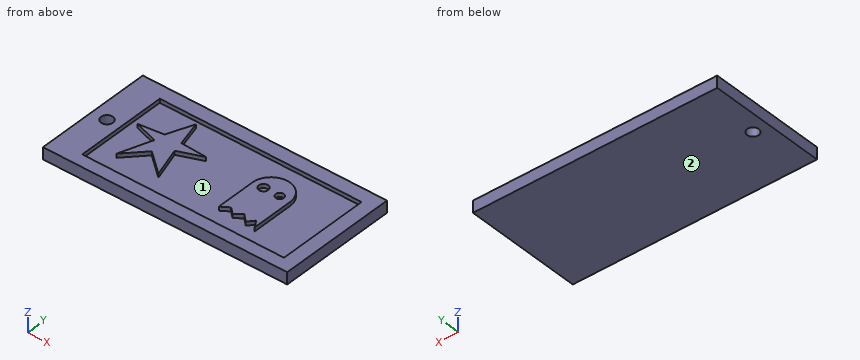
from build123d import *

# Parameters (mm, degrees)
SKETCH_W        = 62
SKETCH_H        = 30
PAD_DEPTH       = 3
SKETCH001_W     = 51.222641
SKETCH001_H     = 23.315135
POCKET_DEPTH    = 1
SKETCH002_R     = 1.5
POCKET001_DEPTH = 3.001
PAD001_DEPTH    = 1
PAD002_DEPTH    = 1
SKETCH005_R     = 1.199553
SKETCH005_R_2   = 1.016367
POCKET002_DEPTH = 1


with BuildPart() as part:
    # Sketch → Pad (new body)
    with BuildSketch(Plane.XY):
        with Locations((-1.286613, 0.704456)):
            Rectangle(SKETCH_W, SKETCH_H)
    extrude(amount=PAD_DEPTH)

    # Sketch001 → Pocket (cut)
    with BuildSketch(Plane.XY.offset(3)):
        with Locations((0.632324, 0.504924)):
            Rectangle(SKETCH001_W, SKETCH001_H)
    extrude(amount=-POCKET_DEPTH, mode=Mode.SUBTRACT)

    # Sketch002 → Pocket001 (cut, through all)
    with BuildSketch(Plane.XY.offset(3)):
        with Locations((-28.453762, 0.41293)):
            Circle(SKETCH002_R)
    extrude(amount=-POCKET001_DEPTH, mode=Mode.SUBTRACT)

    # Sketch003 → Pad001 (new body)
    with BuildSketch(Plane.XY.offset(2)):
        Polygon((-16.856503, 3.99872), (-14.349889, 10.458068), (-12.61454, 3.99872), (-6.058784, 3.709493), (-12.036091, 1.299289), (-9.722297, -6.316956), (-15.313969, -1.689364), (-20.03797, -6.70259), (-17.242132, 1.395697), (-23.123034, 3.227453), align=None)
    extrude(amount=PAD001_DEPTH)

    # Sketch004 → Pad002 (new body)
    with BuildSketch(Plane.XY.offset(2)):
        with BuildLine():
            Line((6.033253, 3.5701), (6.033253, -6.826028))
            Line((6.033253, -6.826028), (8.010232, -5.476315))
            Line((8.010232, -5.476315), (9.649171, -6.922436))
            Line((9.649171, -6.922436), (11.384521, -5.476315))
            Line((11.384521, -5.476315), (13.119864, -7.115253))
            Line((13.119864, -7.115253), (14.469583, -5.572722))
            Line((14.469583, -5.572722), (15.636065, -7.404478))
            Line((15.636065, -7.404478), (15.636065, 3.375676))
            ThreePointArc((15.636065, 3.375676), (10.927253, 8.046213), (6.033253, 3.5701))
        make_face()
    extrude(amount=PAD002_DEPTH)

    # Sketch005 → Pocket002 (cut)
    with BuildSketch(Plane.XY.offset(3)):
        with Locations((8.755972, 3.403389)):
            Circle(SKETCH005_R)
        with Locations((12.882946, 3.403389)):
            Circle(SKETCH005_R_2)
    extrude(amount=-POCKET002_DEPTH, mode=Mode.SUBTRACT)


solid = part.part
The model under review builds one solid part; all positions refer to its coordinate system, in mm. Face numbers are marked on the shaded views. Give positions to 0.01 mm unless a question says otherwise; leave off trailing zeros. Order: outer loops, then holes, each group sorted by start corner. A loop starts at its lowest first (then second) coordinate and runs counter-clockwise, first axis right, second up. Notation, with made-up numbers: M 74,-31 L 86,-31 A27 ccw 86,6 Z; hole C 88,46.25 d11. An arc over 180 degrees is marked long. Answer in a Markdown table with one row per item. Add a question column.
1. Add section C-C on x = 19.5. State the section outline as (y, z) points, plus the area to 3 significant figures.
2. Add section B-B on y = -10. State the section outline as (x, z) points, plus the area to 3 significant figures.
3. Mouldability with a two-part tool opening along X and no side actions: class the marked faces 1 and 2 as released by +X, released by -X, zero draft, split by the parting line, or undercut.
4. For pin 1 Ø1.4 at (x, y) = (8.76, 3.4) entering from +Z, flat-tipped, find the tip position at first contact; note if it passes through.
5. Add section D-D on y = 9. State the section outline as (x, z) points.
6. To check wall thickness, follow line 1 along Y through (x, z) = (22, 2.5); line 2 along Y through (x, z) = (13, 2.05); line 3 along X through (y, z) = (-0.25, 2.15). State the ranges of each line that lie inside material, in increasing order.
7. Add section A-A on z = 2.45. Count the separate pieces of the cut face and the enclosed holes in it, plus the area to 3 significant figures.
The answers:
| question | item | result |
|---|---|---|
| 1 | outline | M -14.3,0 L 15.7,0 L 15.7,3 L 12.16,3 L 12.16,2 L -11.15,2 L -11.15,3 L -14.3,3 Z |
| 1 | area | 66.7 mm2 |
| 2 | outline | M -32.29,0 L 29.71,0 L 29.71,3 L 26.24,3 L 26.24,2 L -24.98,2 L -24.98,3 L -32.29,3 Z |
| 2 | area | 135 mm2 |
| 3 | face 1 | undercut |
| 3 | face 2 | zero draft |
| 4 | pin 1 | z = 2 |
| 5 | outline | M -32.29,0 L 29.71,0 L 29.71,3 L 26.24,3 L 26.24,2 L -13.96,2 L -13.96,3 L -14.92,3 L -14.92,2 L -24.98,2 L -24.98,3 L -32.29,3 Z |
| 6 | line 1 | -14.3 to -11.15, 12.16 to 15.7 |
| 6 | line 2 | -14.3 to -11.15, -7 to 2.39, 4.41 to 7.53, 12.16 to 15.7 |
| 6 | line 3 | -32.29 to -29.8, -27.11 to -24.98, -17.81 to -11.57, 6.03 to 15.64, 26.24 to 29.71 |
| 7 | separate pieces | 3 |
| 7 | enclosed holes | 4 |
| 7 | area | 857 mm2 |
